```python
from build123d import *

# Parameters (mm, degrees)
SKETCH1_W           = 120.675
SKETCH1_H           = 1.5875
SKETCH6_R           = 7.9375
BOSS_EXTRUDE1_DEPTH = 101.6
SKETCH7_R           = 23.308025585
CUT_EXTRUDE3_DEPTH  = 19.075


with BuildPart() as part:
    # Sketch1 → Revolve1 (revolve)
    with BuildSketch(Plane(origin=(0, 0, 0), x_dir=(1, 0, 0), z_dir=(0, 1, 0))):
        with Locations((79.5875, 8.73125)):
            Rectangle(SKETCH1_W, SKETCH1_H)
    revolve(axis=Axis((157.324, 0, 0), (-1, 0, 0)))

    # Sketch6 → Boss-Extrude1 (add)
    with BuildSketch(Plane.ZY.offset(-19.25)):
        with Locations(Location((0, 0, 0), (0, 0, 180))):
            Circle(SKETCH6_R)
    extrude(amount=-BOSS_EXTRUDE1_DEPTH)

    # Sketch7 → Cut-Extrude3 (cut)
    with BuildSketch(Plane(origin=(120.85, 0, 0), x_dir=(0, 0, -1), z_dir=(1, 0, 0))):
        Circle(SKETCH7_R)
    extrude(amount=CUT_EXTRUDE3_DEPTH, mode=Mode.SUBTRACT)


solid = part.part
```
CAD build for the part. Positions are in the model's coordinates, mm. Round coordinates to 2 decimals unless told otherwise and drop trailing zeros. Write each loop counter-clockwise with the first axis right and the second up, starting at its lowest first coordinate (ties: lowest second). Pieces come first, ordered by that corner, then holes. Notation, with made-up numbers: (56, 14) - (70, 14) arc R32 cw to (70, 41) - close; hole circle Ø7 at (7, 48.25). An arc over 180 degrees is marked (long way). Write item = value, one per line. Start each with the question number.
Q1. Band-saw the part on A-A (x = 80). Give the cut face in (y, z) (3 decimals).
Q2. Drop flat-ended pins along their axis: pin 1 (10 mm diameter, centred on x = 110, y = 2, fed in from -Z) (3 decimals); pin 2 (1.5 mm diameter, centred on x = 36, z = -1.5, fed in from -Y); pin 3 (5 mm diameter, centred on x = 46, z = -5.5, fed in from -Y); pin 4 (8 mm diameter, centred on x = 58.5, y = -6.5, fed in from -Z). Give the stop position or say it passes through.
Q3. Band-saw the part on B-B (z = -6). Give the cut face in (x, y), then the cut area to 3 significant figures.
Q4. Band-saw the part on C-C (y = 7.25). Give the cut face in (x, z), then the cut area to 3 significant figures.
Q5. Probe L1, parallel to Z at x = 88, y = -0.25; L2, parallel to Y at x = 63.5, z = -3.5. List the from-to ranges inside material, lowest first. Write a range as from..to.
Answers below:
q1.outline = circle Ø19.05 at (0, 0)
q2.pin_1 = -9.525
q2.pin_2 = -9.5
q2.pin_3 = -9.04
q2.pin_4 = -9.19
q3.outline = (19.25, -7.4) - (120.85, -7.4) - (120.85, 7.4) - (19.25, 7.4) - close
q3.area = 1,500 mm2
q4.outline = (19.25, -6.18) - (120.85, -6.18) - (120.85, 6.18) - (19.25, 6.18) - close
q4.area = 1,260 mm2
q5.L1 = -9.52..9.52
q5.L2 = -8.86..8.86
